Work out the finished part from the listing and answer in its coordinate system (mm). Round coordinates to 2 decimals unless told otherwise and drop trailing zeros. Loops run counter-clockwise (first coordinate to the right, second up) from the corner with the lowest first, then second, coordinate; pieces in that order, holes last. Notation, with made-up numbers: (81, 36.5) - (130, 36.5) arc R29 ccw to (130, 61.5) - close; hole circle Ø6 at (60.5, -33). An arc over 180 degrees is marked (long way). Answer as CSV lines item,"result". Start each with the question number.
Q1. Straight lines are drawn through the part: L1, parallel to X at y = -487.5, z = 251; L2, parallel to X at y = -492.75, z = 221.5. For each, find the intervals that lie inside material, in ascending order. Write a range as [from, to].
Q2. Section B-B on z = 103 is taken. Write down the section's boundary in (x, y), then the cut area to 3 significant figures.
Q3. Section A-A on x = 790 is taken. Count the separate pieces of the cut face and the enclosed holes in it, then the cut area to 3 significant figures.
Q4. Section C-C on z = 214 is taken. Write down the section's boundary in (x, y), then the cut area to 3 significant figures.
Q5. This flat-tipped pin is pushed along its axis until it touches: pin 1 Ø12 at (x, z) = (798.5, 95.5) entering from +Y. Where does it stop, or does it pass through?
Q6. The mould has two halves that part along Z. Classify faces 1 (the face through (784, -495, 26.612)), 2 (the face through (794.299, -495.008, 180.788)), 3 (the face through (780, -484.868, 175)): +Z half, -Z half, draft (parallel to the pull), parting line (faces both ways), or undercut.
```python
from build123d import *

# Parameters (mm, degrees)
SKETCH_W            = 40
SKETCH_H            = 20
PAD_DEPTH           = 300
POCKET_DEPTH        = 12
LINEARPATTERN_COUNT = 15
LINEARPATTERN_PITCH = 21.428571


with BuildPart() as part:
    # Sketch → Pad (new body)
    with BuildSketch(Plane.XY.offset(26.612171)):
        with Locations((0.312673, 1.131631)):
            Rectangle(SKETCH_W, SKETCH_H)
    extrude(amount=PAD_DEPTH)

    # Sketch001 → Pocket (cut, symmetric)
    with BuildSketch(Plane.XZ):
        Polygon((21.003967, 325.206817), (21.003967, 304.575988), (0, 313.960541), align=None)
    pocket = extrude(amount=POCKET_DEPTH, both=True, mode=Mode.SUBTRACT)

    # LinearPattern: Pocket ×15
    with Locations(*[(0, 0, -i * LINEARPATTERN_PITCH) for i in range(1, LINEARPATTERN_COUNT)]):
        add(pocket, mode=Mode.SUBTRACT)


with BuildPart() as part_1:
    # Body placement: moved
    add(part.part.moved(Location((784, -496, 0))))


solid = part_1.part
```
Findings:
1,L1,"x = [764.31, 786.47]"
1,L2,"x = [764.31, 799.1]"
2,outline,"(764.31, -504.87) - (790.21, -504.87) - (790.21, -484.87) - (764.31, -484.87) - close"
2,area,"518 mm^2"
3,separate pieces,"15"
3,enclosed holes,"0"
3,area,"4,350 mm^2"
4,outline,"(764.31, -504.87) - (797.41, -504.87) - (797.41, -484.87) - (764.31, -484.87) - close"
4,area,"662 mm^2"
5,pin 1,"stops at y = -484.87"
6,face 1,"-Z half"
6,face 2,"undercut"
6,face 3,"draft"
